Source: CAD feature listing. Evaluate the final solid. Frame: model axes, mm. Face numbers are marked on the shaded views. A direction names the side the tool comes from. Give positions to 0.01 mm unless a question says otherwise; leave off trailing zeros. Order: outer loops, then holes, each group sorted by start corner. A loop starts at its lowest first (then second) coordinate and runs counter-clockwise, first axis right, second up.
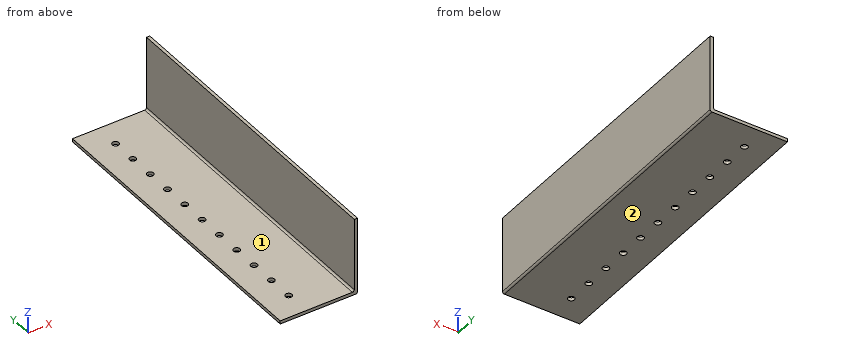
from build123d import *

# Parameters (mm, degrees)
F1_DEPTH = 304.8
F3_R     = 3.175
F4_DEPTH = 76.201


with BuildPart() as f1:
    # F0 (on Front) → F1 (new body)
    with BuildSketch(Plane.XZ):
        with BuildLine():
            Line((-76.2, 0), (-1.8598719395, 0))
            ThreePointArc((-1.8598719395, 0), (-3.5781695574, 1.1481297619), (-3.175, 3.175))
            Line((-3.175, 3.175), (-5.0348719936, 3.175))
            Line((-5.0348719936, 3.175), (-76.2, 3.175))
            Line((-76.2, 3.175), (-76.2, 0))
        make_face()
        with BuildLine():
            ThreePointArc((-3.175, 3.175), (-1.1481297619, 3.5781695574), (0, 1.8598719395))
            Line((0, 1.8598719395), (0, 76.2))
            Line((0, 76.2), (-3.175, 76.2))
            Line((-3.175, 76.2), (-3.175, 5.0348719395))
            Line((-3.175, 5.0348719395), (-3.175, 3.175))
        make_face()
        with BuildLine():
            Line((-5.0348719936, 3.175), (-3.175, 3.175))
            Line((-3.175, 3.175), (-3.175, 5.0348719395))
            ThreePointArc((-3.175, 5.0348719395), (-3.7197438981, 3.7197438598), (-5.0348719936, 3.175))
        make_face()
        with BuildLine():
            ThreePointArc((-3.175, 3.175), (-3.5781695574, 1.1481297619), (-1.8598719395, 0))
            ThreePointArc((-1.8598719395, 0), (-0.5447438789, 0.5447438789), (0, 1.8598719395))
            ThreePointArc((0, 1.8598719395), (-1.1481297619, 3.5781695574), (-3.175, 3.175))
        make_face()
    extrude(amount=F1_DEPTH)

    # F3 (on face) → F4 (cut, through all)
    with BuildSketch(Plane(origin=(0, 0, 0), x_dir=(1, 0, 0), z_dir=(0, 0, -1))):
        with Locations((-50.8, 279.4)):
            Circle(F3_R)
        with Locations((-50.8, 254)):
            Circle(F3_R)
        with Locations((-50.8, 228.6)):
            Circle(F3_R)
        with Locations((-50.8, 203.2)):
            Circle(F3_R)
        with Locations((-50.8, 177.8)):
            Circle(F3_R)
        with Locations((-50.8, 152.4)):
            Circle(F3_R)
        with Locations((-50.8, 127)):
            Circle(F3_R)
        with Locations((-50.8, 101.6)):
            Circle(F3_R)
        with Locations((-50.8, 76.2)):
            Circle(F3_R)
        with Locations((-50.8, 50.8)):
            Circle(F3_R)
        with Locations((-50.8, 25.4)):
            Circle(F3_R)
    extrude(amount=-F4_DEPTH, mode=Mode.SUBTRACT)


solid = f1.part
1) First-contact query: pin 1 Ø12 at (x, z) = (-13, 55.5) entering from +Y; pin 2 Ø7.5 at (x, y) = (-50.8, -50.8) entering from +Z (3 decimals); pin 3 Ø8 at (y, z) = (-122, 12.5) entering from -X (3 decimals). Flat tips, straight axial feed; report the tip coordinate or a pass-through.
Checks:
pin 1: passes through
pin 2: stops at z = 3.175
pin 3: stops at x = -3.175
2) Reachability of the marked faces 1 and 2 from +Z, -Z, +X, -X, +Y, -Y: full face, straight path, thin tool, end or side. Return the list, or none.
Checks:
face 1: +Z, -X, +Y, -Y
face 2: -Z, +X, -X, +Y, -Y
3) Section query A-A on y = -228.6. Output: boundary loops of the cut face in (x, z) (3 decimals), and give its area (3 significant figures).
Checks:
outline: (-76.2, 0) - (-53.975, 0) - (-53.975, 3.175) - (-76.2, 3.175) - close; (-47.625, 0) - (-1.86, 0) arc R1.86 ccw to (0, 1.86) - (0, 76.2) - (-3.175, 76.2) - (-3.175, 5.035) arc R1.86 cw to (-5.035, 3.175) - (-47.625, 3.175) - close
area: 454 mm2
4) Ray query, L1, parallel to X at y = -127, z = 2 (3 decimals); L2, parallel to X at y = -270, z = 12 (3 decimals); L3, parallel to Z at x = -47, y = -256 (3 decimals). Return the intervals inside material, ascending.
Checks:
L1: x = -76.2 to -53.975, -47.625 to 0
L2: x = -3.175 to 0
L3: z = 0 to 3.175
5) Section query C-C on x = -22. Output: boundary loops of the cut face in (y, z) (3 decimals).
Checks:
outline: (-304.8, 0) - (0, 0) - (0, 3.175) - (-304.8, 3.175) - close
6) Section query B-B on z = 34.5. Output: boundary loops of the cut face in (x, y) (3 decimals).
Checks:
outline: (-3.175, -304.8) - (0, -304.8) - (0, 0) - (-3.175, 0) - close
